from build123d import *

# Parameters (mm, degrees)
CUT_EXTRUDE1_REACH          = 110.88
SKETCH5_R                   = 3.175
SKETCH3_W                   = 62.865
SKETCH3_H                   = 71.12
BOSS_EXTRUDE3_DEPTH         = 44.45
SKETCH8_R                   = 22.225
CUT_EXTRUDE3_DEPTH          = 109.879819067
FILLET1_R                   = 2.54
FILLET2_R                   = 2.54
F_1_4_28_TAPPED_HOLE1_D     = 5.4102
F_1_4_28_TAPPED_HOLE1_DEPTH = 12.7
F_1_4_28_TAPPED_HOLE1_TIP   = 1.625388061
F_1_4_28_TAPPED_HOLE7_D     = 5.4102
F_1_4_28_TAPPED_HOLE7_DEPTH = 6.35
F_1_4_28_TAPPED_HOLE8_D     = 5.4102
F_1_4_28_TAPPED_HOLE8_DEPTH = 12.7
F_1_4_28_TAPPED_HOLE8_TIP   = 1.625388061
CUT_EXTRUDE4_DEPTH          = 11.43
CUT_EXTRUDE6_DEPTH          = 9.525
CUT_EXTRUDE6_DEPTH_BACK     = 9.525
F_1_4_28_TAPPED_HOLE9_D     = 5.4102
F_1_4_28_TAPPED_HOLE9_DEPTH = 12.7
F_1_4_28_TAPPED_HOLE9_TIP   = 1.625388061


with BuildPart() as part:
    # Sketch2 → Revolve1 (revolve)
    with BuildSketch(Plane.XY, mode=Mode.PRIVATE) as revolve1_sk:
        Polygon((-22.225, 38.508849789), (-44.45, 38.508849789), (-44.45, 32.158849789), (-28.575, 32.158849789), (-28.575, -44.041150211), (-44.45, -44.041150211), (-44.45, -50.391150211), (-22.225, -50.391150211), (-22.225, 26.465672677), align=None)
    revolve(revolve1_sk.sketch.rotate(Axis((0, -56.084327323, 0), (0, 1, 0)), 270), axis=Axis((0, -56.084327323, 0), (0, 1, 0)))

    # Sketch5 → Cut-Extrude1 (cut, up to next)
    with BuildSketch(Plane(origin=(0, 38.508849789, 0), x_dir=(1, 0, 0), z_dir=(0, 1, 0)), mode=Mode.PRIVATE) as cut_extrude1_sk1:
        with Locations(Location((0, 38.1, 0), (0, 0, 270))):
            Circle(SKETCH5_R)
    cut_extrude1_tool1 = extrude(cut_extrude1_sk1.sketch, amount=-CUT_EXTRUDE1_REACH, mode=Mode.PRIVATE) & part.part
    # Sketch5 → Cut-Extrude1 (cut, up to next)
    with BuildSketch(Plane(origin=(0, 38.508849789, 0), x_dir=(1, 0, 0), z_dir=(0, 1, 0)), mode=Mode.PRIVATE) as cut_extrude1_sk2:
        with Locations(Location((32.995567884, 19.05, 0), (0, 0, 270))):
            Circle(SKETCH5_R)
    cut_extrude1_tool2 = extrude(cut_extrude1_sk2.sketch, amount=-CUT_EXTRUDE1_REACH, mode=Mode.PRIVATE) & part.part
    # Sketch5 → Cut-Extrude1 (cut, up to next)
    with BuildSketch(Plane(origin=(0, 38.508849789, 0), x_dir=(1, 0, 0), z_dir=(0, 1, 0)), mode=Mode.PRIVATE) as cut_extrude1_sk3:
        with Locations(Location((32.995567884, -19.05, 0), (0, 0, 270))):
            Circle(SKETCH5_R)
    cut_extrude1_tool3 = extrude(cut_extrude1_sk3.sketch, amount=-CUT_EXTRUDE1_REACH, mode=Mode.PRIVATE) & part.part
    # Sketch5 → Cut-Extrude1 (cut, up to next)
    with BuildSketch(Plane(origin=(0, 38.508849789, 0), x_dir=(1, 0, 0), z_dir=(0, 1, 0)), mode=Mode.PRIVATE) as cut_extrude1_sk4:
        with Locations(Location((0, -38.1, 0), (0, 0, 270))):
            Circle(SKETCH5_R)
    cut_extrude1_tool4 = extrude(cut_extrude1_sk4.sketch, amount=-CUT_EXTRUDE1_REACH, mode=Mode.PRIVATE) & part.part
    # Sketch5 → Cut-Extrude1 (cut, up to next)
    with BuildSketch(Plane(origin=(0, 38.508849789, 0), x_dir=(1, 0, 0), z_dir=(0, 1, 0)), mode=Mode.PRIVATE) as cut_extrude1_sk5:
        with Locations(Location((-32.995567884, -19.05, 0), (0, 0, 270))):
            Circle(SKETCH5_R)
    cut_extrude1_tool5 = extrude(cut_extrude1_sk5.sketch, amount=-CUT_EXTRUDE1_REACH, mode=Mode.PRIVATE) & part.part
    # Sketch5 → Cut-Extrude1 (cut, up to next)
    with BuildSketch(Plane(origin=(0, 38.508849789, 0), x_dir=(1, 0, 0), z_dir=(0, 1, 0)), mode=Mode.PRIVATE) as cut_extrude1_sk6:
        with Locations(Location((-32.995567884, 19.05, 0), (0, 0, 270))):
            Circle(SKETCH5_R)
    cut_extrude1_tool6 = extrude(cut_extrude1_sk6.sketch, amount=-CUT_EXTRUDE1_REACH, mode=Mode.PRIVATE) & part.part
    add(cut_extrude1_tool1.solids().sort_by_distance((0, 38.50885, -38.1))[0], mode=Mode.SUBTRACT)
    add(cut_extrude1_tool2.solids().sort_by_distance((32.995568, 38.50885, -19.05))[0], mode=Mode.SUBTRACT)
    add(cut_extrude1_tool3.solids().sort_by_distance((32.995568, 38.50885, 19.05))[0], mode=Mode.SUBTRACT)
    add(cut_extrude1_tool4.solids().sort_by_distance((0, 38.50885, 38.1))[0], mode=Mode.SUBTRACT)
    add(cut_extrude1_tool5.solids().sort_by_distance((-32.995568, 38.50885, 19.05))[0], mode=Mode.SUBTRACT)
    add(cut_extrude1_tool6.solids().sort_by_distance((-32.995568, 38.50885, -19.05))[0], mode=Mode.SUBTRACT)

    # Sketch3 → Boss-Extrude3 (add)
    with BuildSketch(Plane(origin=(44.45, 0, 0), x_dir=(0, 0, -1), z_dir=(1, 0, 0))):
        with Locations((0, 2.948849789)):
            Rectangle(SKETCH3_W, SKETCH3_H)
    extrude(amount=-BOSS_EXTRUDE3_DEPTH)

    # Sketch8 → Cut-Extrude3 (cut, through all)
    with BuildSketch(Plane(origin=(0, 38.508849789, 0), x_dir=(1, 0, 0), z_dir=(0, 1, 0))):
        with Locations(Location((0, 0, 0), (0, 0, 90))):
            Circle(SKETCH8_R)
    extrude(amount=-CUT_EXTRUDE3_DEPTH, mode=Mode.SUBTRACT)

    # Fillet1
    fillet1_edges = [part.edges().sort_by_distance(p)[0] for p in [
        (0, -0.226150211, -31.4325),
        (0, -0.226150211, 31.4325),
    ]]
    fillet(fillet1_edges, radius=FILLET1_R)

    # Fillet2
    # the kernel refuses this fillet: 2.54 mm, written as the material it adds along each edge
    with BuildSketch(Plane(origin=(0, 32.158849789, 0), x_dir=(0.22074631689702245, 0, -0.9753312583816841), z_dir=(0.9753312583816841, 0, 0.22074631689702245))) as fillet2_piece_1:
        with BuildLine():
            CenterArc((28.575 + FILLET2_R, -FILLET2_R), FILLET2_R, 90, 90)
            Line((28.575, -FILLET2_R), (28.575, 0))
            Line((28.575, 0), (28.575 + FILLET2_R, 0))
        make_face()
    revolve(axis=Axis((0, 32.158849789, 0), (0, 1, 0)), revolution_arc=205.505743093)
    with BuildSketch(Plane(origin=(0, -44.041150211, 0), x_dir=(0, 0, -1), z_dir=(1, 0, 0))) as fillet2_piece_2:
        with BuildLine():
            CenterArc((28.575 + FILLET2_R, FILLET2_R), FILLET2_R, 180, 90)
            Line((28.575 + FILLET2_R, 0), (28.575, 0))
            Line((28.575, 0), (28.575, FILLET2_R))
        make_face()
    revolve(axis=Axis((0, -44.041150211, 0), (0, 1, 0)))

    # 1/4-28 Tapped Hole1
    with Locations(Plane(origin=(44.45, 32.158849789, 12.7), x_dir=(0, 0, 1), z_dir=(1, 0, 0))):
        with Locations((0, 0), (-25.4, 0), (-38.1, 6.985), (-38.1, 29.21), (-38.1, 51.435), (-25.4, 58.42), (0, 58.42)):
            Hole(F_1_4_28_TAPPED_HOLE1_D / 2, depth=F_1_4_28_TAPPED_HOLE1_DEPTH)
            with Locations((0, 0, -(F_1_4_28_TAPPED_HOLE1_DEPTH + F_1_4_28_TAPPED_HOLE1_TIP / 2))):  # 118° drill point
                Cone(0, F_1_4_28_TAPPED_HOLE1_D / 2, F_1_4_28_TAPPED_HOLE1_TIP, mode=Mode.SUBTRACT)

    # 1/4-28 Tapped Hole7
    with Locations(Plane(origin=(0, -50.391150211, -37.949057556), x_dir=(0, 0, -1), z_dir=(0, -1, 0))):
        with Locations((0, 0), (-25.249057556, 35.760886026), (-50.649057556, 35.760886026), (-25.249057556, -35.760886026), (-50.649057556, -35.760886026), (-75.898115112, 0)):
            Hole(F_1_4_28_TAPPED_HOLE7_D / 2, depth=F_1_4_28_TAPPED_HOLE7_DEPTH)

    # 1/4-28 Tapped Hole8
    with Locations(Plane(origin=(32.995567884, 38.508849789, -19.05), x_dir=(0, 0, 1), z_dir=(0, 1, 0))):
        with Locations((0, 0), (38.1, 0)):
            Hole(F_1_4_28_TAPPED_HOLE8_D / 2, depth=F_1_4_28_TAPPED_HOLE8_DEPTH)
            with Locations((0, 0, -(F_1_4_28_TAPPED_HOLE8_DEPTH + F_1_4_28_TAPPED_HOLE8_TIP / 2))):  # 118° drill point
                Cone(0, F_1_4_28_TAPPED_HOLE8_D / 2, F_1_4_28_TAPPED_HOLE8_TIP, mode=Mode.SUBTRACT)

    # Sketch13 → Cut-Extrude4 (cut)
    with BuildSketch(Plane(origin=(44.45, 0, 0), x_dir=(0, 0, -1), z_dir=(1, 0, 0))):
        with BuildLine():
            Line((9.525, 14.061349789), (-9.525, 14.061349789))
            ThreePointArc((-9.525, 14.061349789), (-11.1125, 12.473849789), (-9.525, 10.886349789))
            Line((-9.525, 10.886349789), (9.525, 10.886349789))
            ThreePointArc((9.525, 10.886349789), (11.1125, 12.473849789), (9.525, 14.061349789))
        make_face()
        with BuildLine():
            Line((7.4295, 6.631849789), (-7.4295, 6.631849789))
            ThreePointArc((-7.4295, 6.631849789), (-11.1125, 2.948849789), (-7.4295, -0.734150211))
            Line((-7.4295, -0.734150211), (7.4295, -0.734150211))
            ThreePointArc((7.4295, -0.734150211), (11.1125, 2.948849789), (7.4295, 6.631849789))
        make_face()
        with BuildLine():
            Line((-9.525, -8.163650211), (9.525, -8.163650211))
            ThreePointArc((9.525, -8.163650211), (11.1125, -6.576150211), (9.525, -4.988650211))
            Line((9.525, -4.988650211), (-9.525, -4.988650211))
            ThreePointArc((-9.525, -4.988650211), (-11.1125, -6.576150211), (-9.525, -8.163650211))
        make_face()
    extrude(amount=-CUT_EXTRUDE4_DEPTH, mode=Mode.SUBTRACT)

    # Sketch22 → Cut-Extrude6 (cut, two sides: drawn at the far end of the back side and taken through both)
    with BuildSketch(Plane.XY.offset(-CUT_EXTRUDE6_DEPTH_BACK)):
        Polygon((33.02, 14.061349789), (22.118863764, 33.487032124), (22.118863764, 36.643703979), (34.791433783, 14.061349789), align=None)
        Polygon((33.02, -8.163650211), (22.118863764, -46.84942144), (22.118863764, -51.230401207), (34.25450188, -8.163650211), align=None)
    extrude(amount=CUT_EXTRUDE6_DEPTH + CUT_EXTRUDE6_DEPTH_BACK, mode=Mode.SUBTRACT)

    # 1/4-28 Tapped Hole9
    with Locations(Plane(origin=(44.45, -12.926150211, 25.4), x_dir=(0, 0, 1), z_dir=(1, 0, 0))):
        with Locations((0, 0), (0, -31.75)):
            Hole(F_1_4_28_TAPPED_HOLE9_D / 2, depth=F_1_4_28_TAPPED_HOLE9_DEPTH)
            with Locations((0, 0, -(F_1_4_28_TAPPED_HOLE9_DEPTH + F_1_4_28_TAPPED_HOLE9_TIP / 2))):  # 118° drill point
                Cone(0, F_1_4_28_TAPPED_HOLE9_D / 2, F_1_4_28_TAPPED_HOLE9_TIP, mode=Mode.SUBTRACT)


solid = part.part
Verification items for the finished model (mm, model axes). A direction names the side the tool comes from. Coordinates: 2 decimals unless noted, no trailing zeros. One line per item, written item: value. Start each with the question number.
Item 1: Gauge pin test, flat ends, axial feed: pin 1 (3 mm diameter, centred on x = 8, y = -26.5, fed in from -Z); pin 2 (5 mm diameter, centred on y = 2.95, z = -25.4, fed in from -X); pin 3 (6 mm diameter, centred on x = -3.5, y = -21.5, fed in from -Z). Record the tip position at first contact, or that the pin passes through.
Item 2: Scan lines: probe 1 along Y at (x, z) = (39.25, 25.4); probe 2 along Y at (x, z) = (31.5, 29.5); probe 3 along Y at (x, z) = (39, -12). Record each from-to range of solid material in increasing order.
Item 3: Sectioned sample at A-A (y = -30.5). Count the separate pieces of the cut face and the enclosed holes in it, then the cut area to 3 significant figures.
Item 4: Mould release check, pull along Y, two halves, no side actions. Record for faces 1 (the flat face through (9.3, -50.391, 20.4)), 2 (the cylindrical face through (-33.93, -47.17, 10.71)), 3 (the flat face through (33.02, 12, 0)), 4 (the conical face through (30.407, 2.808, -24.952)): released by +Y, released by -Y, zero draft, split by the parting line, or undercut.
Item 5: Access from +Z, -Z, +X, -X, +Y, -Y to the whole of each face (thin tool, end or side, straight path). Record for faces 5 (the flat face through (39, -8.164, 0)), 6 (the flat face through (-29, 32.159, -13)), 7 (the cylindrical face through (37.589, -47.172, -14.694)).
Conclusion:
1. pin 1: stops at z = -31.43
1. pin 2: stops at x = -17.09
1. pin 3: stops at z = -28.57
2. probe 1: y = -32.61 to -15.63, -10.22 to 16.12, 21.53 to 38.51
2. probe 2: y = -50.39 to -44.04, -32.61 to 38.51
2. probe 3: y = -50.39 to -44.04, -32.61 to -28.87, -23.65 to 29.55, 34.77 to 38.51
3. separate pieces: 1
3. enclosed holes: 2
3. area: 2,500 mm^2
4. face 1: released by -Y
4. face 2: zero draft
4. face 3: undercut
4. face 4: undercut
5. face 5: +X
5. face 6: -X
5. face 7: -Y
